```python
from build123d import *

# Parameters (mm, degrees)
EXTRUDE_1_DEPTH      = 3.175
EXTRUDE_1_DEPTH_BACK = 3.175
SKETCH_1_R           = 31.75
SKETCH_1_R_2         = 25.4
SKETCH_2_R           = 29.3878
SKETCH_2_R_2         = 27.7622
CUT_EXTRUDE_1_DEPTH  = 0.254


with BuildPart() as part:
    # Sketch 1 → Extrude 1 (new, two sides: drawn at the far end of the back side and taken through both)
    with BuildSketch(Plane(origin=(0, 0, 0), x_dir=(1, 0, 0), z_dir=(0, 1, 0)).offset(-EXTRUDE_1_DEPTH_BACK)):
        with Locations(Location((0, 0, 0), (0, 0, 270))):
            Circle(SKETCH_1_R)
        with Locations(Location((0, 0, 0), (0, 0, 270))):
            Circle(SKETCH_1_R_2, mode=Mode.SUBTRACT)
    extrude(amount=EXTRUDE_1_DEPTH + EXTRUDE_1_DEPTH_BACK)

    # Sketch 2 → Cut-Extrude 1 (cut)
    with BuildSketch(Plane(origin=(0, 3.175, 0), x_dir=(1, 0, 0), z_dir=(0, 1, 0))):
        with Locations(Location((0, 0, 0), (0, 0, 270))):
            Circle(SKETCH_2_R)
        with Locations(Location((0, 0, 0), (0, 0, 270))):
            Circle(SKETCH_2_R_2, mode=Mode.SUBTRACT)
    cut_extrude_1 = extrude(amount=-CUT_EXTRUDE_1_DEPTH, mode=Mode.SUBTRACT)

    # Mirror 1: Cut-Extrude 1 across plane
    add(cut_extrude_1.mirror(Plane.ZX), mode=Mode.SUBTRACT)


solid = part.part
```
Part model, mm, in its own coordinate system. A direction names the side the tool comes from. Coordinates: 2 decimals unless noted, no trailing zeros. Write each loop counter-clockwise with the first axis right and the second up, starting at its lowest first coordinate (ties: lowest second). Pieces come first, ordered by that corner, then holes.
Item 1: Pin check, flat tips, straight feed: pin 1 (1 mm diameter, centred on x = 5, y = -0.5, fed in from +Z); pin 2 (3 mm diameter, centred on x = -22, y = 2.5, fed in from -Z); pin 3 (1 mm diameter, centred on y = 2.5, z = -17.5, fed in from -X). Stop position of each tip, or through.
Item 2: Slice it at C-C (y = -0.75). Write the cut outline in (x, z), and give its area (3 significant figures).
Item 3: Slice it at B-B (z = 0). Write the cut outline in (x, y) (3 decimals).
Item 4: Probe line 1 (X direction, y = 3, z = 0); line 2 (Z direction, x = -19, y = -0.5); line 3 (X direction, y = 0.5, z = 14). List the from-to ranges inside material, lowest first.
Item 5: Mould opens along X. For faces 1 (the face through (-30.995, -0.044, -6.883)), 2 (the face through (-22.5, 3.175, 12.2)), 3 (the face through (-15.456, -0.044, -20.157)) say: released by +X, released by -X, zero draft, split by the parting line, or undercut.
Item 6: Slice it at A-A (x = 0). Write the cut outline in (y, z) (3 decimals).
Item 7: Which spindle directions (+Z, -Z, +X, -X, +Y, -Y) get a long thin tool onto all of the face, cutting with end or side? Do faces 4 (the face through (18, 2.921, 22)), 5 (the face through (18, -2.921, 22)), 6 (the face through (-9.3, -3.175, 28.1)). Say none if no direction does.
Results found:
1. pin 1: stops at z = 31.43
1. pin 2: stops at z = -24.24
1. pin 3: stops at x = -26.82
2. outline: circle Ø63.5 at (0, 0); hole circle Ø50.8 at (0, 0)
2. area: 1,140 mm2
3. outline: (-31.75, -3.175) - (-29.388, -3.175) - (-29.388, -2.921) - (-27.762, -2.921) - (-27.762, -3.175) - (-25.4, -3.175) - (-25.4, 3.175) - (-27.762, 3.175) - (-27.762, 2.921) - (-29.388, 2.921) - (-29.388, 3.175) - (-31.75, 3.175) - close; (25.4, -3.175) - (27.762, -3.175) - (27.762, -2.921) - (29.388, -2.921) - (29.388, -3.175) - (31.75, -3.175) - (31.75, 3.175) - (29.388, 3.175) - (29.388, 2.921) - (27.762, 2.921) - (27.762, 3.175) - (25.4, 3.175) - close
4. line 1: x = -31.75 to -29.39, -27.76 to -25.4, 25.4 to 27.76, 29.39 to 31.75
4. line 2: z = -25.44 to -16.86, 16.86 to 25.44
4. line 3: x = -28.5 to -21.19, 21.19 to 28.5
5. face 1: split by the parting line
5. face 2: zero draft
5. face 3: undercut
6. outline: (-3.175, -31.75) - (3.175, -31.75) - (3.175, -29.388) - (2.921, -29.388) - (2.921, -27.762) - (3.175, -27.762) - (3.175, -25.4) - (-3.175, -25.4) - (-3.175, -27.762) - (-2.921, -27.762) - (-2.921, -29.388) - (-3.175, -29.388) - close; (-3.175, 25.4) - (3.175, 25.4) - (3.175, 27.762) - (2.921, 27.762) - (2.921, 29.388) - (3.175, 29.388) - (3.175, 31.75) - (-3.175, 31.75) - (-3.175, 29.388) - (-2.921, 29.388) - (-2.921, 27.762) - (-3.175, 27.762) - close
7. face 4: +Y
7. face 5: -Y
7. face 6: +Z, -Z, +X, -X, -Y
